```python
from build123d import *

# Parameters (mm, degrees)
REVOLVE1_ANGLE      = 30
SKETCH2_R           = 7.14375
BOSS_EXTRUDE1_DEPTH = 2.54
SKETCH3_R           = 7.14375
BOSS_EXTRUDE2_DEPTH = 6.35
SKETCH4_W           = 34.925
SKETCH4_H           = 20.32
CUT_REVOLVE1_ANGLE  = 30


with BuildPart() as part:
    # Sketch1 → Revolve1 (revolve)
    with BuildSketch(Plane.XY):
        Polygon((-43.4975, 0), (-43.4975, 2.54), (-42.2275, 2.54), (-42.2275, 17.78), (-43.4975, 17.78), (-43.4975, 20.32), (-39.6875, 20.32), (-39.6875, 0), align=None)
    revolve(axis=Axis((0, 0, 0), (0, 1, 0)), revolution_arc=REVOLVE1_ANGLE)

    # Sketch2 → Boss-Extrude1 (add)
    with BuildSketch(Plane(origin=(-37.028941606, 0, 9.921875), x_dir=(0.258819045, 0, 0.965925826), z_dir=(-0.965925826, 0, 0.258819045))):
        with Locations((0, 10.16)):
            Circle(SKETCH2_R)
    extrude(amount=BOSS_EXTRUDE1_DEPTH)

    # Sketch3 → Boss-Extrude2 (add)
    with BuildSketch(Plane(origin=(-37.028941606, 0, 9.921875), x_dir=(-0.258819045, 0, -0.965925826), z_dir=(0.965925826, 0, -0.258819045))):
        with Locations((0, 10.16)):
            Circle(SKETCH3_R)
    extrude(amount=BOSS_EXTRUDE2_DEPTH)

    # Sketch4 → Cut-Revolve1 (revolve, cut)
    with BuildSketch(Plane.XY):
        with Locations((-17.4625, 10.16)):
            Rectangle(SKETCH4_W, SKETCH4_H)
    revolve(axis=Axis((0, 0, 0), (0, 1, 0)), revolution_arc=CUT_REVOLVE1_ANGLE, mode=Mode.SUBTRACT)


solid = part.part
```
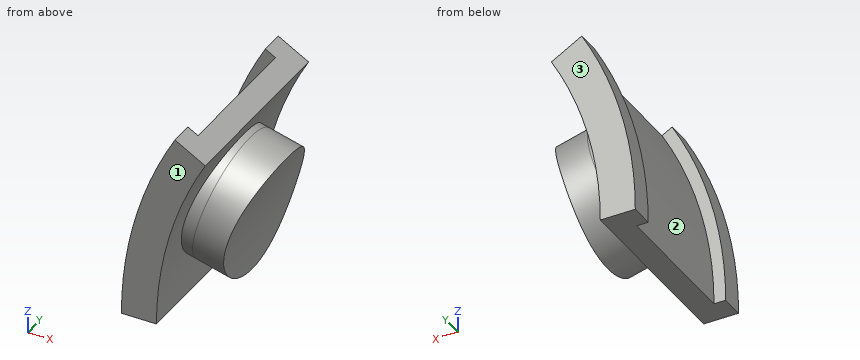
Could you check a few things on this model? Use its own coordinates, in mm. Face numbers are marked on the shaded views. Give positions to 0.01 mm unless a question says otherwise; leave off trailing zeros. Write each loop counter-clockwise with the first axis right and the second up, starting at its lowest first coordinate (ties: lowest second). Pieces come first, ordered by that corner, then holes. Notation, with made-up numbers: (-8.75, 42) - (37.25, 42) arc R18 cw to (37.25, 69) - close; hole circle Ø10 at (-17.75, 35). An arc over 180 degrees is marked (long way). One line per item, written item: value. Start each with the question number.
Item 1: Imagine slicing it at A-A, the plane x = -41.75. List the corners of the cut face in (y, z) for me, and give its area (3 significant figures).
Item 2: If we mould it in two halves opening along Y, with no side actions, what happens to the marked faces 1, 2 and 3? For each: +Y half, -Y half, draft (parallel to the pull), parting line (faces both ways), or undercut.
Item 3: I'm going to push flat-ended pins straight in: pin 1 (1.5 mm diameter, centred on y = 4, z = 19.5, fed in from +X); pin 2 (6 mm diameter, centred on y = 17.5, z = 8, fed in from +X); pin 3 (5 mm diameter, centred on x = -42, z = 19, fed in from +Y). Where does each tip first touch, or does it pass through?
Item 4: Please list where these lines run through material, in increasing order: line 1 (Y direction, x = -38.25, z = 18); line 2 (Z direction, x = -35.25, y = 14); line 3 (Z direction, x = -35.5, y = 7). Write a range as from..to.
Geometry says:
1. outline: (0, 0) - (20.32, 0) - (20.32, 12.21) - (17.78, 12.21) - (17.78, 6.33) - (2.54, 6.33) - (2.54, 12.21) - (0, 12.21) - close
1. area: 159 mm^2
2. face 1: -Y half
2. face 2: undercut
2. face 3: +Y half
3. pin 1: x = -34.37
3. pin 2: x = -33.16
3. pin 3: through
4. line 1: 0..2.54, 17.78..20.32
4. line 2: 3.21..15.68, 18.24..20.35
4. line 3: 2.88..16.15, 17.74..20.5
